```python
from build123d import *

# Parameters (mm, degrees)
SKETCH_1_R        = 20
EXTRUDE_1_DEPTH   = 50
EXTRUDE_1_2_DEPTH = 25


with BuildPart() as part:
    # 草图1 → Extrude 1 (new body)
    with BuildSketch(Plane.XY):
        Circle(SKETCH_1_R)
    extrude(amount=EXTRUDE_1_DEPTH)

    # 草图3 → Extrude 1 2 (add, symmetric)
    with BuildSketch(Plane(origin=(0, 0, 0), x_dir=(1, 0, 0), z_dir=(0, 1, 0))):
        Polygon((20, 0), (-27.7557358, -36.128356044), (-27.761769046, -36.120381086), (19.993966754, 0.007974957), align=None)
    extrude(amount=EXTRUDE_1_2_DEPTH, both=True)


solid = part.part
```
CAD build for the part. Positions are in the model's coordinates, mm. Coordinates: 2 decimals unless noted, no trailing zeros. Use a Markdown table: item, result. Add a question column.
(1) Drill centre lines: line 1 along Z through (x, y) = (-2, -15.5); line 2 along Y through (x, z) = (13, 26); line 3 along X through (y, z) = (-2, 5). Where is each one in solid material? Low to high. Write a range as [from, to].
(2) Flat gauge pins, fed straight in: pin 1 (6 mm diameter, centred on y = 15, z = 23.5, fed in from -X); pin 2 (10 mm diameter, centred on x = -0.5, z = 27.5, fed in from +Y); pin 3 (2 mm diameter, centred on x = -5, z = 29.5, fed in from -Y). Where does each tip first touch, or does it go through?
(3) Pull direction X, two halves, no side cores. Call faces 1 (the face through (0, 0, 0)), 2 (the face through (19.076, 6.007, 30.206)): +X half, -X half, draft (parallel to the pull), parting line (faces both ways), or undercut.
Solved:
| question | item | result |
|---|---|---|
| 1 | line 1 | z = [0, 50] |
| 1 | line 2 | y = [-15.2, 15.2] |
| 1 | line 3 | x = [-19.9, 19.9] |
| 2 | pin 1 | stops at x = -16 |
| 2 | pin 2 | stops at y = 20 |
| 2 | pin 3 | stops at y = -19.6 |
| 3 | face 1 | draft |
| 3 | face 2 | undercut |
